Check sheet for the modelled part. Datum: model origin and axes. Units: mm. Face numbers are marked on the shaded views. Coordinates: 2 decimals unless noted, no trailing zeros. Write each loop counter-clockwise with the first axis right and the second up, starting at its lowest first coordinate (ties: lowest second). Pieces come first, ordered by that corner, then holes. Notation, with made-up numbers: M -18,28.5 L 41,28.5 A14 cw 41,49.5 Z; hole C 48.5,26 d7. An arc over 180 degrees is marked long. Answer as CSV lines item,"result". Start each with the question number.
1) Section check D-D (z = 7). Record the cut outline in (x, y), and give its area (3 significant figures).
2) Section check C-C (z = 72). Record the cut outline in (x, y).
3) Draft check along Y on the marked faces 1, 2 and 3. Enter one of: +Y half, -Y half, draft (parallel to the pull), parting line (faces both ways), or undercut.
4) Material ranges on L1, parallel to Z at x = 20, y = 6 (3 decimals); L2, parallel to Y at x = 0, z = 27.5; L3, parallel to X at y = 9, z = 29.5, recorded low to high. Write a range as [from, to].
5) Section check A-A (x = 0). Record the cut outline in (y, z) (3 decimals).
6) Go/stop test with flat-tipped pins: pin 1 Ø1 at (x, z) = (10.5, 45.5) entering from +Y; pin 2 Ø12 at (y, z) = (12.5, 47) entering from -X; pin 3 Ø4 at (y, z) = (-12.5, 41.5) entering from +X; pin 4 Ø10 at (x, y) = (5, -20) entering from -Z. Record where each tip stops, or that it passes through.
from build123d import *

# Parameters (mm, degrees)
ESQUISSE1_R             = 25.099999965
BOSS_EXTRU_1_DEPTH      = 57.15
ESQUISSE2_R             = 21.25
ENL_V_MAT_EXTRU_1_DEPTH = 53.975
ESQUISSE3_R             = 5.565233599
BOSS_EXTRU_2_DEPTH      = 25.4
CONG_1_R                = 2
CONG_2_R                = 2


with BuildPart() as part:
    # Esquisse1 → Boss.-Extru.1 (new body)
    with BuildSketch(Plane.XY):
        Circle(ESQUISSE1_R)
    extrude(amount=BOSS_EXTRU_1_DEPTH)

    # Esquisse2 → Enlèv. mat.-Extru.1 (cut)
    with BuildSketch(Plane(origin=(0, 0, 0), x_dir=(-1, 0, 0), z_dir=(0, 0, -1))):
        Circle(ESQUISSE2_R)
    extrude(amount=-ENL_V_MAT_EXTRU_1_DEPTH, mode=Mode.SUBTRACT)

    # Esquisse3 → Boss.-Extru.2 (add)
    with BuildSketch(Plane.XY.offset(57.15)):
        Circle(ESQUISSE3_R)
    extrude(amount=BOSS_EXTRU_2_DEPTH)

    # Congé1
    cong_1_edges = [part.edges().sort_by_distance(p)[0] for p in [
        (21.25, 0, 0),
    ]]
    fillet(cong_1_edges, radius=CONG_1_R)

    # Congé2
    cong_2_edges = [part.edges().sort_by_distance(p)[0] for p in [
        (-5.565233599, 0, 57.15),
    ]]
    fillet(cong_2_edges, radius=CONG_2_R)

    # Esquisse4 → Enlèvement de matière-Révolution1 (revolve, cut)
    with BuildSketch(Plane(origin=(0, 0, 0), x_dir=(0, 0, -1), z_dir=(1, 0, 0)), mode=Mode.PRIVATE) as enl_vement_de_mati_re_r_volution1_sk:
        with BuildLine():
            Line((-57.15, 25.099999965), (0, 25.099999965))
            ThreePointArc((0, 25.099999965), (-28.575, 23.487538039), (-57.15, 25.099999965))
        make_face()
    revolve(enl_vement_de_mati_re_r_volution1_sk.sketch.rotate(Axis((0, 0, 82.55), (0, 0, -1)), 90), axis=Axis((0, 0, 82.55), (0, 0, -1)), mode=Mode.SUBTRACT)


solid = part.part
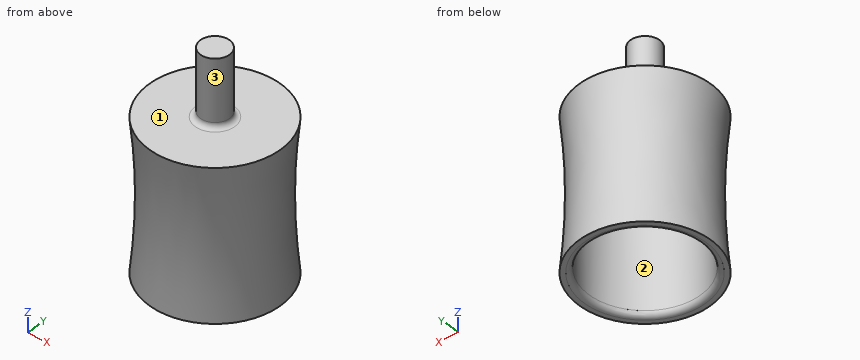
Results found:
1,outline,"C 0,0 d48.81; hole C 0,0 d42.5"
1,area,"453 mm2"
2,outline,"C 0,0 d11.13"
3,face 1,"draft"
3,face 2,"undercut"
3,face 3,"parting line"
4,L1,"z = [53.975, 57.15]"
4,L2,"y = [-23.49, -21.25], [21.25, 23.49]"
4,L3,"x = [-21.7, -19.25], [19.25, 21.7]"
5,outline,"M -25.1,0 L -23.25,0 A2 ccw -21.25,2 L -21.25,53.975 L 21.25,53.975 L 21.25,2 A2 ccw 23.25,0 L 25.1,0 A254 cw 25.1,57.15 L 7.565,57.15 A2 cw 5.565,59.15 L 5.565,82.55 L -5.565,82.55 L -5.565,59.15 A2 cw -7.565,57.15 L -25.1,57.15 A254 cw Z"
6,pin 1,"stops at y = 21.88"
6,pin 2,"stops at x = -23.33"
6,pin 3,"stops at x = 21.38"
6,pin 4,"stops at z = 0"
